from build123d import *

# Parameters (mm, degrees)
EXTRUDE_306_DEPTH          = 25
CUT_EXTRUDE_407_DEPTH      = 26.735837529
CUT_EXTRUDE_407_DEPTH_BACK = 26.735837529
SKETCH_8_R                 = 5.5
SKETCH_8_R_2               = 4.5


with BuildPart() as part:
    # 草图1 → Extrude 306 (new, symmetric)
    with BuildSketch(Plane(origin=(0, 0, 0), x_dir=(0, 0, -1), z_dir=(1, 0, 0))):
        Polygon((4.618802154, 0), (2.309401077, 4), (-2.309401077, 4), (-4.618802154, 0), (-2.309401077, -4), (2.309401077, -4), align=None)
    extrude(amount=EXTRUDE_306_DEPTH, both=True)

    # 草图8 → Cut-Extrude 407 (cut, two sides: drawn at the far end of the back side and taken through both)
    with BuildSketch(Plane(origin=(0, 0, 0), x_dir=(0, 0, -1), z_dir=(1, 0, 0)).offset(-CUT_EXTRUDE_407_DEPTH_BACK)):
        Circle(SKETCH_8_R)
        Circle(SKETCH_8_R_2, mode=Mode.SUBTRACT)
    extrude(amount=CUT_EXTRUDE_407_DEPTH + CUT_EXTRUDE_407_DEPTH_BACK, mode=Mode.SUBTRACT)

    # 草图10 → Cut-Revolve 698 (revolve, cut)
    with BuildSketch(Plane.XY, mode=Mode.PRIVATE) as cut_revolve_698_sk:
        Polygon((-25.5, 4.5), (-24, 4.5), (-25.5, 3), align=None)
        Polygon((24, 4.5), (25.5, 3), (25.5, 4.5), align=None)
    revolve(cut_revolve_698_sk.sketch.rotate(Axis((25, 0, 0), (-1, 0, 0)), 267.266044451), axis=Axis((25, 0, 0), (-1, 0, 0)), mode=Mode.SUBTRACT)


solid = part.part
Geometry check sheet. Reference: the model listing, model coordinates, mm. Give positions to 0.01 mm unless a question says otherwise; leave off trailing zeros. Order: outer loops, then holes, each group sorted by start corner. A loop starts at its lowest first (then second) coordinate and runs counter-clockwise, first axis right, second up.
1) Cross-section at A-A (x = -17.5). Record the boundary of the cut face in (y, z).
Results are:
outline: (-4, -2.06) arc R4.5 ccw to (-3.79, -2.43) - (-0.21, -4.49) arc R4.5 ccw to (0.21, -4.49) - (3.79, -2.43) arc R4.5 ccw to (4, -2.06) - (4, 2.06) arc R4.5 ccw to (3.79, 2.43) - (0.21, 4.49) arc R4.5 ccw to (-0.21, 4.49) - (-3.79, 2.43) arc R4.5 ccw to (-4, 2.06) - close
2) Gauge pin test, flat end, axial feed: pin 1 (3 mm diameter, centred on x = 8, y = 2.5, fed in from +Z). Record the tip position at first contact, or that the pin passes through.
Results are:
pin 1: stops at z = 4.04
3) Material ranges on probe 1 along Z at (x, y) = (5.5, -1); probe 2 along X at (y, z) = (-0.5, -3.5); probe 3 along X at (y, z) = (3.75, -1.75), recorded low to high.
Results are:
probe 1: z = -4.04 to 4.04
probe 2: x = -24.96 to 24.96
probe 3: x = -24.36 to 24.36
